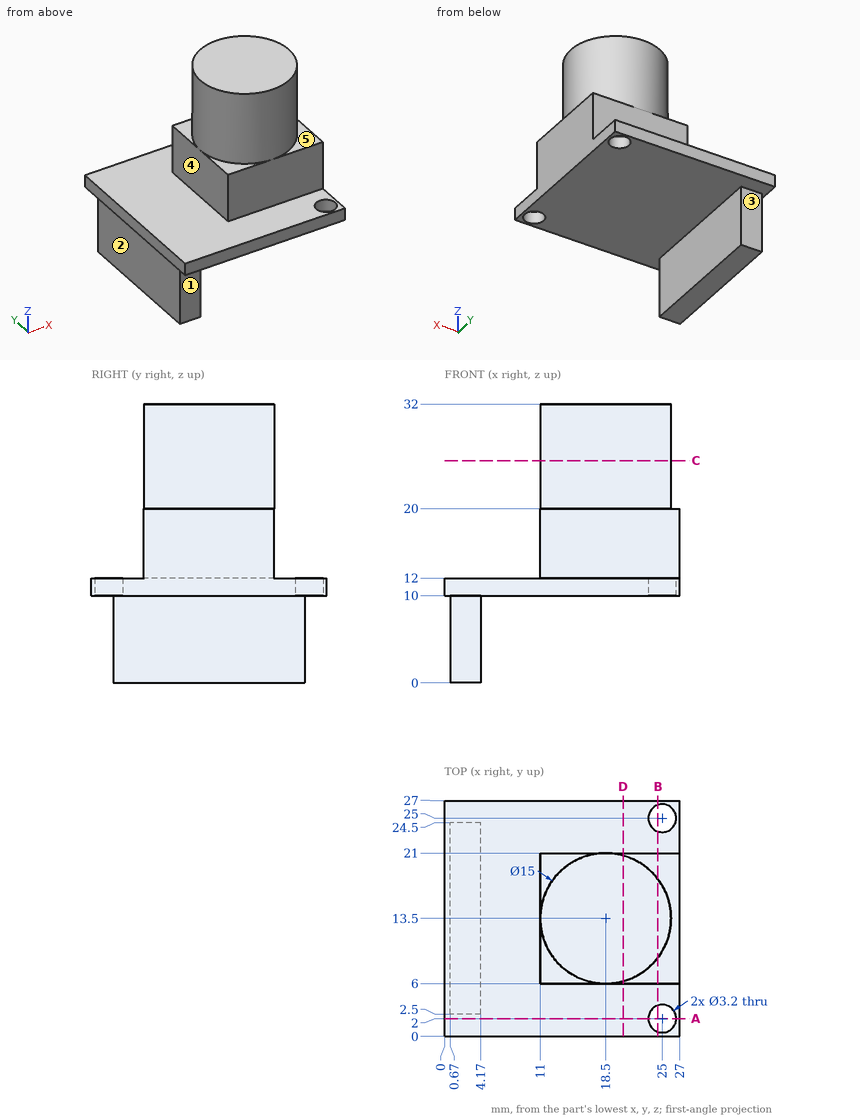
Check sheet for the drawn part. Datum: minimum x, y, z corner. Units: mm. A direction names the side the tool comes from. Coordinates: 2 decimals unless noted, no trailing zeros. Loops run counter-clockwise (first coordinate to the right, second up) from the corner with the lowest first, then second, coordinate; pieces in that order, holes last. Notation, with made-up numbers: (40.5, 38.5) - (44.5, 38.5) arc R22 cw to (44.5, 62.5) - close; hole circle Ø1 at (63.5, 38). An arc over 180 degrees is marked (long way). Put each result on its own line as item: value.
Item 1: Section check A-A (y = 2). Enter the section's corners in (x, z).
Conclusion:
outline: (0, 10) - (23.4, 10) - (23.4, 12) - (0, 12) - close; (26.6, 10) - (27, 10) - (27, 12) - (26.6, 12) - close
Item 2: Scan lines: line 1 along Y through (x, z) = (25, 11.55); line 2 along X through (y, z) = (25, 10.9); line 3 along Z through (x, y) = (13.75, 15.5). Record each from-to range of solid material in increasing order.
Conclusion:
line 1: y = 0 to 0.4, 3.6 to 23.4, 26.6 to 27
line 2: x = 0 to 23.4, 26.6 to 27
line 3: z = 10 to 32
Item 3: Set-up check for the marked faces 1, 2, 3, 4 and 5: record each of +Z, -Z, +X, -X, +Y, -Y from which the full face is reachable in a straight line by a thin tool's end or side.
Conclusion:
face 1: -Z, +X, -X, -Y
face 2: -Z, -X, +Y, -Y
face 3: -Z, +X, -X, +Y
face 4: +Z, -X, +Y, -Y
face 5: +Z, +X
Item 4: Section check D-D (x = 20.5). Enter the section's corners in (y, z), then the cut area to 3 significant figures.
Conclusion:
outline: (0, 10) - (27, 10) - (27, 12) - (21, 12) - (21, 20) - (20.73, 20) - (20.73, 32) - (6.27, 32) - (6.27, 20) - (6, 20) - (6, 12) - (0, 12) - close
area: 347 mm2
Item 5: Section check B-B (x = 24.5). Enter the section's corners in (y, z).
Conclusion:
outline: (0, 10) - (0.48, 10) - (0.48, 12) - (0, 12) - close; (3.52, 10) - (23.48, 10) - (23.48, 12) - (21, 12) - (21, 20) - (18, 20) - (18, 32) - (9, 32) - (9, 20) - (6, 20) - (6, 12) - (3.52, 12) - close; (26.52, 10) - (27, 10) - (27, 12) - (26.52, 12) - close
Item 6: Gauge pin test, flat ends, axial feed: pin 1 Ø1.5 at (y, z) = (19.5, 8) entering from -X; pin 2 Ø8 at (y, z) = (4.5, 27.5) entering from +X; pin 3 Ø8 at (x, y) = (13, 12) entering from -Z; pin 4 Ø3 at (x, y) = (25, 2) entering from -Z. Record the tip position at first contact, or that the pin passes through.
Conclusion:
pin 1: stops at x = 0.67
pin 2: stops at x = 24.09
pin 3: stops at z = 10
pin 4: passes through
Item 7: Section check C-C (z = 25.5). Enter the section's corners in (x, y).
Conclusion:
outline: circle Ø15 at (18.5, 13.5)
